from build123d import *

# Parameters (mm, degrees)
SKETCH_1_W          = 48
SKETCH_1_H          = 30
EXTRUDE_1_DEPTH     = 65
SKETCH_2_R          = 15
EXTRUDE_2_DEPTH     = 6.75
EXTRUDE_START       = 6.75
SKETCH_3_R          = 15
EXTRUDE_3_DEPTH     = 6.75
SKETCH_4_R          = 1.25
SKETCH_4_R_2        = 5
CUT_EXTRUDE_1_DEPTH = 87.299261295
SKETCH_5_R          = 5
CUT_EXTRUDE_2_DEPTH = 33
SKETCH_6_R          = 5
EXTRUDE_4_DEPTH     = 10


with BuildPart() as part:
    # 草图1 → 凸台-拉伸1 (new body)
    with BuildSketch(Plane.XY):
        Rectangle(SKETCH_1_W, SKETCH_1_H)
    extrude(amount=EXTRUDE_1_DEPTH)

    # 草图2 → 凸台-拉伸2 (add)
    with BuildSketch(Plane.ZY.offset(24)):
        with Locations(Location((13, 0, 0), (0, 0, 270))):
            Circle(SKETCH_2_R)
    extrude(amount=EXTRUDE_2_DEPTH)

    # 草图3 → 凸台-拉伸3 (add)
    with BuildSketch(Plane(origin=(24, 0, 0), x_dir=(0, 0, -1), z_dir=(1, 0, 0)).offset(EXTRUDE_START)):
        with Locations(Location((-13, 0, 0), (0, 0, 270))):
            Circle(SKETCH_3_R)
    extrude(amount=-EXTRUDE_3_DEPTH)

    # 草图4 → 切除-拉伸1 (cut, through all)
    with BuildSketch(Plane(origin=(24, 0, 0), x_dir=(0, 0, -1), z_dir=(1, 0, 0))):
        with Locations(Location((-62, 12, 0), (0, 0, 90))):
            Circle(SKETCH_4_R)
        with Locations(Location((-38, 12, 0), (0, 0, 90))):
            Circle(SKETCH_4_R)
        with Locations(Location((-38, -12, 0), (0, 0, 90))):
            Circle(SKETCH_4_R)
        with Locations(Location((-62, -12, 0), (0, 0, 90))):
            Circle(SKETCH_4_R)
        with Locations(Location((-50, 12, 0), (0, 0, 90))):
            Circle(SKETCH_4_R)
        with Locations(Location((-50, -12, 0), (0, 0, 90))):
            Circle(SKETCH_4_R)
        with Locations(Location((-62, 0, 0), (0, 0, 90))):
            Circle(SKETCH_4_R)
        with Locations(Location((-50, 0, 0), (0, 0, 90))):
            Circle(SKETCH_4_R_2)
    extrude(amount=-CUT_EXTRUDE_1_DEPTH, mode=Mode.SUBTRACT)

    # 草图5 → 切除-拉伸2 (cut)
    with BuildSketch(Plane.XZ.offset(15)):
        with Locations((0, 55)):
            Circle(SKETCH_5_R)
    extrude(amount=-CUT_EXTRUDE_2_DEPTH, mode=Mode.SUBTRACT)

    # 草图6 → 凸台-拉伸4 (add)
    with BuildSketch(Plane.XY.offset(65)):
        Circle(SKETCH_6_R)
    extrude(amount=-EXTRUDE_4_DEPTH)


solid = part.part
Here's how the part is built. I have some questions about the finished solid (model axes, mm). A direction names the side the tool comes from. Coordinates: 2 decimals unless noted, no trailing zeros. Order: outer loops, then holes, each group sorted by start corner. A loop starts at its lowest first (then second) coordinate and runs counter-clockwise, first axis right, second up. Notation, with made-up numbers: (-26, 72) -> (3, 72) arc R18 cw to (3, 82) -> close; hole circle Ø7 at (41.5, 86.25). An arc over 180 degrees is marked (long way). Answer in a Markdown table with one row per item.
(1) Will these pins go through, and if not, where does the flat tip stop? pin 1 Ø3 at (y, z) = (0, 62) entering from -X; pin 2 Ø2 at (y, z) = (12, 50) entering from -X; pin 3 Ø1 at (x, y) = (23.5, 8) entering from -Z; pin 4 Ø4 at (y, z) = (-12, 62) entering from +X.
Answer key:
| item | result |
|---|---|
| pin 1 | x = -24 |
| pin 2 | through |
| pin 3 | z = 0 |
| pin 4 | x = 24 |
(2) I want a section at D-D on z = 25. List the corners of the cut face in (x, y) for me.
Answer key:
| item | result |
|---|---|
| outline | (-30.75, -9) -> (-24, -9) -> (-24, -15) -> (24, -15) -> (24, -9) -> (30.75, -9) -> (30.75, 9) -> (24, 9) -> (24, 15) -> (-24, 15) -> (-24, 9) -> (-30.75, 9) -> close |
(3) I want a section at A-A on x = 0. List the corners of the cut face in (y, z) for me, then the cut area to 3 significant figures.
Answer key:
| item | result |
|---|---|
| outline | (-15, 0) -> (15, 0) -> (15, 50) -> (13.25, 50) arc R1.25 cw to (10.75, 50) -> (5, 50) arc R5 cw to (-5, 50) -> (-10.75, 50) arc R1.25 cw to (-13.25, 50) -> (-15, 50) -> close; (-15, 60) -> (-5, 60) -> (-5, 55) -> (5, 55) -> (5, 60) -> (15, 60) -> (15, 65) -> (-15, 65) -> close; hole circle Ø2.5 at (-12, 38); hole circle Ø2.5 at (-12, 62); hole circle Ø2.5 at (12, 38); hole circle Ø2.5 at (12, 62) |
| area | 1,640 mm^2 |
(4) I want a section at C-C on y = 12. List the corners of the cut face in (x, z) for me, then the cut area to 3 significant figures.
Answer key:
| item | result |
|---|---|
| outline | (-30.75, 4) -> (-24, 4) -> (-24, 0) -> (24, 0) -> (24, 4) -> (30.75, 4) -> (30.75, 22) -> (24, 22) -> (24, 36.75) -> (-24, 36.75) -> (-24, 22) -> (-30.75, 22) -> close; (-24, 39.25) -> (24, 39.25) -> (24, 48.75) -> (-24, 48.75) -> close; (-24, 51.25) -> (-3.31, 51.25) arc R5 cw (long way) to (3.31, 51.25) -> (24, 51.25) -> (24, 60.75) -> (-24, 60.75) -> close; (-24, 63.25) -> (24, 63.25) -> (24, 65) -> (-24, 65) -> close |
| area | 2,930 mm^2 |
(5) Please list where these lines run through material, in increasing order: probe 1 along Z at (x, y) = (13, 0); probe 2 along Z at (x, y) = (-8, -12); probe 3 along Z at (x, y) = (-4, -13).
Answer key:
| item | result |
|---|---|
| probe 1 | 0 to 45, 55 to 60.75, 63.25 to 65 |
| probe 2 | 0 to 36.75, 39.25 to 48.75, 51.25 to 60.75, 63.25 to 65 |
| probe 3 | 0 to 37.25, 38.75 to 49.25, 50.75 to 52, 58 to 61.25, 62.75 to 65 |
(6) On a 3-axis mill with a long thin cutter (end or side, diameter ignored), from which of +Z, -Z, +X, -X, +Y, -Y can I reach the whole of each face in a straight line? I mean faces 1 (the face through (24, 0, -1)), 2 (the face through (24, -13, 3)), 3 (the face through (-24, 13, 3)). Say none if no direction works.
Answer key:
| item | result |
|---|---|
| face 1 | -Z, +Y, -Y |
| face 2 | -Z, +X, -Y |
| face 3 | -Z, -X, +Y |
(7) Thinking about a two-plate mould opening in Z: for faces 4 (the face through (5, 0, 62)), 5 (the face through (-24, 0, -1)), 6 (the face through (-27.328, 1.953, 27.872)), which applies, +Z half, -Z half, draft (parallel to the pull), parting line (faces both ways), or undercut?
Answer key:
| item | result |
|---|---|
| face 4 | undercut |
| face 5 | draft |
| face 6 | parting line |
(8) I want a section at B-B on z = 62. List the corners of the cut face in (x, y) for me, then the cut area to 3 significant figures.
Answer key:
| item | result |
|---|---|
| outline | (-24, -15) -> (24, -15) -> (24, -13.25) -> (-24, -13.25) -> close; (-24, -10.75) -> (24, -10.75) -> (24, -1.25) -> (4.84, -1.25) arc R5 ccw to (4.84, 1.25) -> (24, 1.25) -> (24, 10.75) -> (-24, 10.75) -> (-24, 1.25) -> (-4.84, 1.25) arc R5 ccw to (-4.84, -1.25) -> (-24, -1.25) -> close; (-24, 13.25) -> (24, 13.25) -> (24, 15) -> (-24, 15) -> close |
| area | 1,100 mm^2 |
